The figure shows three views and two pictorial views of one solid part (mm, origin at its lowest corner). Answer the questions. A direction names the side the tool comes from. Give positions to 0.01 mm unless a question says otherwise; leave off trailing zeros. Loops run counter-clockwise (first coordinate to the right, second up) from the corner with the lowest first, then second, coordinate; pieces in that order, holes last. Notation, with made-up numbers: M 86.5,59.5 L 134.5,59.5 A18 cw 134.5,91.5 Z; hole C 68.5,17.5 d7. An arc over 180 degrees is marked long. Answer as a JSON object with one key per item and string values. Group by question number.
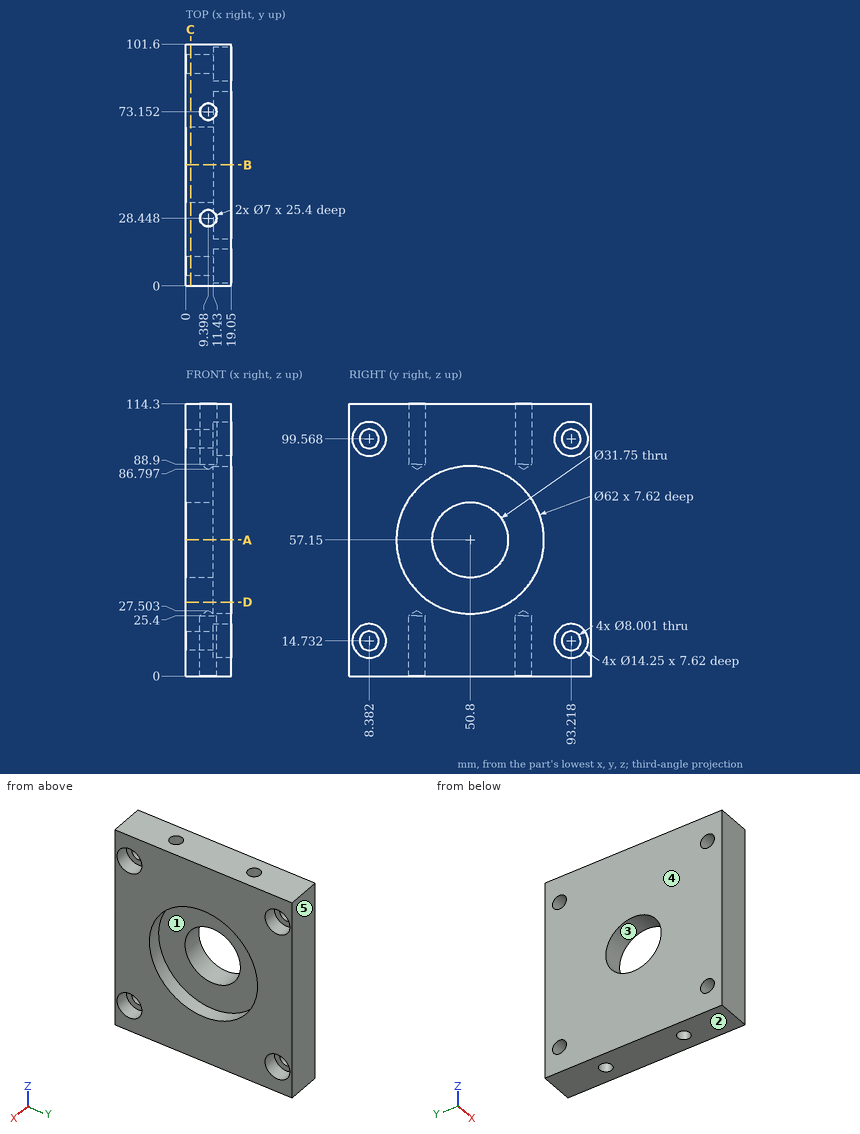
Item 1: A tool of negligible diameter and unlimited length cuts with its end or side. For the marked faces 1 and 2, from which of +Z, -Z, +X, -X, +Y, -Y can it reach the whole face along a straight path? Write none if from no direction.
Item 2: Find the intervals of material crossed by probe 1 along Z at (x, y) = (16.75, 8); probe 2 along Y at (x, z) = (2.75, 98.5); probe 3 along Y at (x, z) = (17, 104.5), in increasing order. Write a range as [from, to].
Item 3: A cutting plane is placed at B-B (y = 50.8). Determine the outline of the cut face in (x, z) (3 decimals).
Item 4: For a pull along Y with two mould halves and no side action, classify the marked faces 3, 4 and 5 as pulls with the +Y half, pulls with the -Y half, needs draft (parallel to the pull), parting line crosses it, or undercut.
Item 5: A cutting plane is placed at A-A (z = 57.15). Determine the outline of the cut face in (x, y) (3 decimals).
Item 6: A cutting plane is placed at D-D (z = 31). Determine the outline of the cut face in (x, y), and give its area (3 significant figures).
Item 7: Given pin 1 Ø16.5 at (y, z) = (8.382, 99.568) entering from -X; pin 2 Ø13 at (y, z) = (93.218, 14.732) entering from +X; pin 3 Ø4 at (x, y) = (9.398, 73.152) entering from -Z; pin 4 Ø1.5 at (y, z) = (91, 101) entering from -X, each flat-ended and moving along its own axis, determine where each tip first touches the part or whether it passes through.
Item 8: A cutting plane is placed at C-C (x = 2). Give the number of separate pieces and of enclosed holes in the cut face, and give its area (3 significant figures).
The answers:
{
 "1": {"face 1": "+X", "face 2": "-Z, +X, -X, +Y, -Y"},
 "2": {"probe 1": "z = [0, 7.62], [21.85, 92.45], [106.68, 114.3]", "probe 2": "y = [0, 4.53], [12.24, 89.36], [97.07, 101.6]", "probe 3": "y = [0, 3.24], [13.52, 88.08], [98.36, 101.6]"},
 "3": {"outline": "M 0,0 L 19.05,0 L 19.05,26.15 L 11.43,26.15 L 11.43,41.275 L 0,41.275 Z; M 0,73.025 L 11.43,73.025 L 11.43,88.15 L 19.05,88.15 L 19.05,114.3 L 0,114.3 Z"},
 "4": {"face 3": "undercut", "face 4": "needs draft", "face 5": "pulls with the +Y half"},
 "5": {"outline": "M 0,0 L 19.05,0 L 19.05,19.8 L 11.43,19.8 L 11.43,34.925 L 0,34.925 Z; M 0,66.675 L 11.43,66.675 L 11.43,81.8 L 19.05,81.8 L 19.05,101.6 L 0,101.6 Z"},
 "6": {"outline": "M 0,0 L 19.05,0 L 19.05,34.15 L 11.43,34.15 L 11.43,67.45 L 19.05,67.45 L 19.05,101.6 L 0,101.6 Z", "area": "1,680 mm^2"},
 "7": {"pin 1": "stops at x = 0", "pin 2": "stops at x = 11.43", "pin 3": "stops at z = 26.3", "pin 4": "passes through"},
 "8": {"separate pieces": "1", "enclosed holes": "5", "area": "10,600 mm^2"}
}
